Geometry: final body of the model. Coordinates: model frame, mm. Face numbers are marked on the shaded views. Give positions to 0.01 mm unless a question says otherwise; leave off trailing zeros. Loops run counter-clockwise (first coordinate to the right, second up) from the corner with the lowest first, then second, coordinate; pieces in that order, holes last.
1. Material intervals for line 1 along Y through (x, z) = (-15, -15.5); line 2 along Y through (x, z) = (-15, -10); line 3 along X through (y, z) = (195, -17), sorted ascending.
2. Draft query along Y for the marked faces 1 and 2. Return one class per face: +Y half, -Y half, draft (parallel to the pull), parting line (faces both ways), or undercut.
3. Section B-B, the plane y = 33. Output: boundary loops of the cut face in (x, z), then the cut area to 3 significant figures.
4. Section A-A, the plane z = 28.5. Output: boundary loops of the cut face in (x, y), then the cut area to 3 significant figures.
5. First-contact query: P1, Ø2, axis at x = -10, y = -153, coming from the +Z side; P2, Ø9.5, axis at x = -15, y = 195, coming from the -Z side; P3, Ø15, axis at x = -21, z = -2, coming from the +Y side; P4, Ø2, axis at x = -16, z = -14.5, coming from the +Y side. Flat tips, straight axial feed; report the tip coordinate or a pass-through.
from build123d import *

# Parameters (mm, degrees)
F0_W      = 490
F0_H      = 43
F1_DEPTH  = 30
F2_R      = 4
F3_DEPTH  = 16
F4_SIZE   = 1
F5_R      = 4
F6_DEPTH  = 16
F7_SIZE   = 1
F8_R      = 3
F9_R      = 6
F10_DEPTH = 15
F11_R     = 4
F12_DEPTH = 16
F13_SIZE  = 1


with BuildPart() as f1:
    # F0 (on Right) → F1 (new body)
    with BuildSketch(Plane.YZ):
        Rectangle(F0_W, F0_H)
    extrude(amount=-F1_DEPTH)

    # F2 (on face) → F3 (join)
    with BuildSketch(Plane(origin=(0, 245, 0), x_dir=(-1, 0, 0), z_dir=(0, 1, 0))):
        with Locations((15, 9.5)):
            Circle(F2_R)
        with Locations((15, -9.5)):
            Circle(F2_R)
    extrude(amount=F3_DEPTH)

    # F4
    f4_edges = [f1.edges().sort_by_distance(p)[0] for p in [
        (-11, 261, 9.5),
        (-11, 261, -9.5),
    ]]
    chamfer(f4_edges, length=F4_SIZE)

    # F5 (on face) → F6 (join)
    with BuildSketch(Plane.XZ.offset(245)):
        with Locations((-15, 9.5)):
            Circle(F5_R)
        with Locations((-15, -9.5)):
            Circle(F5_R)
    extrude(amount=F6_DEPTH)

    # F7
    f7_edges = [f1.edges().sort_by_distance(p)[0] for p in [
        (-19, -261, 9.5),
        (-19, -261, -9.5),
    ]]
    chamfer(f7_edges, length=F7_SIZE)

    # F8
    f8_edges = [f1.edges().sort_by_distance(p)[0] for p in [
        (-30, 0, -21.5),
        (0, 0, -21.5),
    ]]
    fillet(f8_edges, radius=F8_R)

    # F9 (on face) → F10 (cut)
    with BuildSketch(Plane(origin=(0, 0, -21.5), x_dir=(1, 0, 0), z_dir=(0, 0, -1))):
        with Locations((-15, 195)):
            Circle(F9_R)
        with Locations((-15, 0)):
            Circle(F9_R)
        with Locations((-15, -195)):
            Circle(F9_R)
    extrude(amount=-F10_DEPTH, mode=Mode.SUBTRACT)

    # F11 (on face) → F12 (join)
    with BuildSketch(Plane.XY.offset(21.5)):
        with Locations((-15, 195)):
            Circle(F11_R)
        with Locations((-15, 0)):
            Circle(F11_R)
        with Locations((-15, -195)):
            Circle(F11_R)
    extrude(amount=F12_DEPTH)

    # F13
    f13_edges = [f1.edges().sort_by_distance(p)[0] for p in [
        (-19, 195, 37.5),
        (-19, 0, 37.5),
        (-19, -195, 37.5),
    ]]
    chamfer(f13_edges, length=F13_SIZE)


solid = f1.part
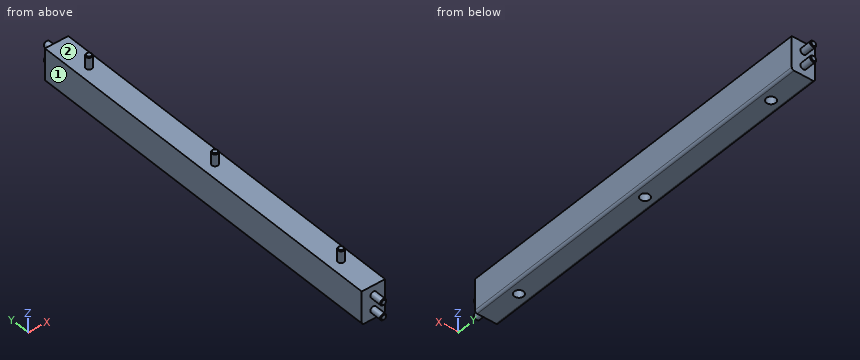
Answers below:
1. line 1: y = -245 to -201, -189 to -6, 6 to 189, 201 to 245
1. line 2: y = -261 to -201, -189 to -6, 6 to 189, 201 to 261
1. line 3: x = -30 to -21, -9 to 0
2. face 1: draft
2. face 2: undercut
3. outline: (-30, -18.5) arc R3 ccw to (-27, -21.5) - (-3, -21.5) arc R3 ccw to (0, -18.5) - (0, 21.5) - (-30, 21.5) - close
3. area: 1,290 mm2
4. outline: circle Ø8 at (-15, -195); circle Ø8 at (-15, 0); circle Ø8 at (-15, 195)
4. area: 151 mm2
5. P1: stops at z = 21.5
5. P2: stops at z = -6.5
5. P3: stops at y = 261
5. P4: stops at y = 245
